Model file for the job. Use its own axes, mm. A direction names the side the tool comes from. Coordinates: 2 decimals unless noted, no trailing zeros. Order: outer loops, then holes, each group sorted by start corner. A loop starts at its lowest first (then second) coordinate and runs counter-clockwise, first axis right, second up.
from build123d import *

# Parameters (mm, degrees)
SKETCH1_W           = 19.5
SKETCH1_H           = 10
BOSS_EXTRUDE1_DEPTH = 4
SKETCH2_W           = 9
SKETCH2_H           = 5.5
CUT_EXTRUDE1_DEPTH  = 2.7
SKETCH3_W           = 3.2
SKETCH3_H           = 3.9
CUT_EXTRUDE2_DEPTH  = 12.664583147
SKETCH4_W           = 1.747901038
SKETCH4_H           = 5.5
CUT_EXTRUDE3_DEPTH  = 12.285056491
CHAMFER2_SIZE       = 1
SKETCH5_W           = 10
SKETCH5_H           = 4
BOSS_EXTRUDE2_DEPTH = 2
SKETCH6_W           = 1.747077863
SKETCH6_H           = 5.5
BOSS_EXTRUDE3_DEPTH = 1.5
BOSS_EXTRUDE4_DEPTH = 2
BOSS_EXTRUDE5_REACH = 16.109
SKETCH9_W           = 3.657403566
SKETCH9_H           = 0.3
SKETCH10_W          = 5.81497097
SKETCH10_H          = 2.25
SKETCH10_W_2        = 5.452409629
BOSS_EXTRUDE6_DEPTH = 2
SKETCH11_W          = 2.603359148
SKETCH11_H          = 5.5
BOSS_EXTRUDE7_DEPTH = 3.8
CHAMFER3_SIZE       = 0.5
SKETCH12_W          = 10
SKETCH12_H          = 6
CUT_EXTRUDE4_DEPTH  = 3.8


with BuildPart() as part:
    # Sketch1 → Boss-Extrude1 (new body)
    with BuildSketch(Plane(origin=(0, 0, 0), x_dir=(1, 0, 0), z_dir=(0, 1, 0))):
        Rectangle(SKETCH1_W, SKETCH1_H)
    extrude(amount=BOSS_EXTRUDE1_DEPTH)

    # Sketch2 → Cut-Extrude1 (cut)
    with BuildSketch(Plane(origin=(0, 4, 0), x_dir=(1, 0, 0), z_dir=(0, 1, 0))):
        with Locations((5.25, 0)):
            Rectangle(SKETCH2_W, SKETCH2_H)
    extrude(amount=-CUT_EXTRUDE1_DEPTH, mode=Mode.SUBTRACT)

    # Sketch3 → Cut-Extrude2 (cut, through all)
    with BuildSketch(Plane(origin=(0, 4, 0), x_dir=(1, 0, 0), z_dir=(0, 1, 0))):
        with Locations((-8.15, 3.05)):
            Rectangle(SKETCH3_W, SKETCH3_H)
        with Locations((-8.15, -3.05)):
            Rectangle(SKETCH3_W, SKETCH3_H)
    extrude(amount=-CUT_EXTRUDE2_DEPTH, mode=Mode.SUBTRACT)

    # Sketch4 → Cut-Extrude3 (cut, through all)
    with BuildSketch(Plane(origin=(0, 1.3, 0), x_dir=(1, 0, 0), z_dir=(0, 1, 0))):
        with Locations((1.623950519, 0)):
            Rectangle(SKETCH4_W, SKETCH4_H)
    extrude(amount=-CUT_EXTRUDE3_DEPTH, mode=Mode.SUBTRACT)

    # Chamfer2
    chamfer2_edges = [part.edges().sort_by_distance(p)[0] for p in [
        (2.497901038, 1.3, 0),
    ]]
    chamfer(chamfer2_edges, length=CHAMFER2_SIZE)

    # Sketch5 → Boss-Extrude2 (add)
    with BuildSketch(Plane(origin=(9.75, 0, 0), x_dir=(0, 0, -1), z_dir=(1, 0, 0))):
        with Locations((0, 2)):
            Rectangle(SKETCH5_W, SKETCH5_H)
    extrude(amount=BOSS_EXTRUDE2_DEPTH)

    # Sketch6 → Boss-Extrude3 (add)
    with BuildSketch(Plane(origin=(0, 1.3, 0), x_dir=(1, 0, 0), z_dir=(0, 1, 0))):
        with Locations((8.876461068, 0)):
            Rectangle(SKETCH6_W, SKETCH6_H)
    extrude(amount=BOSS_EXTRUDE3_DEPTH)

    # Sketch7 → Boss-Extrude4 (add)
    with BuildSketch(Plane(origin=(0, 4, 0), x_dir=(1, 0, 0), z_dir=(0, 1, 0))):
        Polygon((2.760699465, 2.75), (2.760699465, 5), (11.75, 5), (11.75, -5), (2.760699465, -5), (2.760699465, -2.75), (9.75, -2.75), (9.75, 2.75), align=None)
    extrude(amount=BOSS_EXTRUDE4_DEPTH)

    # Sketch9 → Boss-Extrude5 (add, up to next)
    with BuildSketch(Plane(origin=(0, 6, 0), x_dir=(1, 0, 0), z_dir=(0, 1, 0)), mode=Mode.PRIVATE) as boss_extrude5_sk1:
        with Locations((7.921298217, 2.6)):
            Rectangle(SKETCH9_W, SKETCH9_H)
    boss_extrude5_tool1 = extrude(boss_extrude5_sk1.sketch, amount=-BOSS_EXTRUDE5_REACH, mode=Mode.PRIVATE) - part.part
    # Sketch9 → Boss-Extrude5 (add, up to next)
    with BuildSketch(Plane(origin=(0, 6, 0), x_dir=(1, 0, 0), z_dir=(0, 1, 0)), mode=Mode.PRIVATE) as boss_extrude5_sk2:
        with Locations((7.921298217, -2.6)):
            Rectangle(SKETCH9_W, SKETCH9_H)
    boss_extrude5_tool2 = extrude(boss_extrude5_sk2.sketch, amount=-BOSS_EXTRUDE5_REACH, mode=Mode.PRIVATE) - part.part
    add(boss_extrude5_tool1.solids().sort_by_distance((7.921298, 6, -2.6))[0])
    add(boss_extrude5_tool2.solids().sort_by_distance((7.921298, 6, 2.6))[0])

    # Sketch10 → Boss-Extrude6 (add)
    with BuildSketch(Plane(origin=(0, 4, 0), x_dir=(1, 0, 0), z_dir=(0, 1, 0))):
        with Locations((-3.642514515, 3.875)):
            Rectangle(SKETCH10_W, SKETCH10_H)
        with Locations((-3.823795186, -3.875)):
            Rectangle(SKETCH10_W_2, SKETCH10_H)
    extrude(amount=BOSS_EXTRUDE6_DEPTH)

    # Sketch11 → Boss-Extrude7 (add)
    with BuildSketch(Plane(origin=(0, 4, 0), x_dir=(1, 0, 0), z_dir=(0, 1, 0))):
        with Locations((-5.248320426, 0)):
            Rectangle(SKETCH11_W, SKETCH11_H)
    extrude(amount=BOSS_EXTRUDE7_DEPTH)

    # Chamfer3
    chamfer3_edges = [part.edges().sort_by_distance(p)[0] for p in [
        (-5.248320426, 7.8, 2.75),
        (-5.248320426, 7.8, -2.75),
    ]]
    chamfer(chamfer3_edges, length=CHAMFER3_SIZE)

    # Sketch12 → Cut-Extrude4 (cut)
    with BuildSketch(Plane.ZY.offset(6.55)):
        with Locations((0, 3)):
            Rectangle(SKETCH12_W, SKETCH12_H)
    extrude(amount=CUT_EXTRUDE4_DEPTH, mode=Mode.SUBTRACT)


solid = part.part
Q1. Probe line 1 (Z direction, x = -1.75, y = 5.5); line 2 (X direction, y = 5.25, z = -0.75); line 3 (X direction, y = 2.5, z = 0.75). List the from-to ranges inside material, lowest first.
Established:
line 1: z = -5 to -2.75, 2.75 to 5
line 2: x = -6.55 to -3.95, 9.75 to 11.75
line 3: x = -6.55 to 0.75, 8 to 11.75
Q2. Drop flat-ended pins along their axis: P1, Ø0.6, axis at x = -5.5, y = 6.5, coming from the +Z side; P2, Ø1.8, axis at x = -3, z = 4, coming from the +Y side; P3, Ø1.4, axis at x = 6, z = 1, coming from the +Y side. Give the stop position or say it passes through.
Established:
P1: stops at z = 2.75
P2: stops at y = 6
P3: stops at y = 1.3
Q3. Cut at C-C, the plane y = 3.5. List the corners of the cut face in (x, z), plus the area to 3 significant figures.
Established:
outline: (-6.55, -5) - (11.75, -5) - (11.75, 5) - (-6.55, 5) - close; hole (0.75, -2.75) - (6.09, -2.75) - (6.09, -2.45) - (9.75, -2.45) - (9.75, 2.45) - (6.09, 2.45) - (6.09, 2.75) - (0.75, 2.75) - close
area: 136 mm2
Q4. Mould opens along X. For faces 4 (the face through (2, 3, 5)), 5 (the face through (-3, 5, 2.75)) say: pulls with the +X half, pulls with the -X half, needs draft (parallel to the pull), parting line crosses it, or undercut.
Established:
face 4: needs draft
face 5: undercut
Q5. Which spindle directions (+Z, -Z, +X, -X, +Y, -Y) get a long thin tool onto all of the face, cutting with end or side? Do faces 1 (the face through (-3.947, 6, 0)), 2 (the face through (-4, 6, -4)), 3 (the face through (2.761, 5, -4)). Say none if no direction does.
Established:
face 1: +Y
face 2: -Z, +X, -X, +Y
face 3: +Z, -Z, +Y
Q6. Cut at B-B, the plane x = 5.75. List the corners of the cut face in (y, z), plus the area to 4 significant figures.
Established:
outline: (0, -5) - (6, -5) - (6, -2.75) - (1.3, -2.75) - (1.3, 2.75) - (6, 2.75) - (6, 5) - (0, 5) - close
area: 34.15 mm2
Q7. Cut at D-D, the plane x = -3.25. List the corners of the cut face in (y, z), plus the area to 3 significant figures.
Established:
outline: (0, -5) - (6, -5) - (6, -2.75) - (4, -2.75) - (4, 2.75) - (6, 2.75) - (6, 5) - (0, 5) - close
area: 49.0 mm2
Q8. Cut at A-A, the plane y = 2. List the corners of the cut face in (x, z), plus the area to 3 significant figures.
Established:
outline: (-6.55, -5) - (11.75, -5) - (11.75, 5) - (-6.55, 5) - close; hole (0.75, -2.75) - (6.09, -2.75) - (6.09, -2.45) - (8, -2.45) - (8, 2.45) - (6.09, 2.45) - (6.09, 2.75) - (0.75, 2.75) - close
area: 144 mm2
